Input: dimensioned drawing with shaded views. Units: mm. Origin: part minimum x, y, z. Give positions to 0.01 mm unless a question says otherwise; leave off trailing zeros. Order: outer loops, then holes, each group sorted by start corner. A loop starts at its lowest first (then second) coordinate and runs counter-clockwise, first axis right, second up. Notation, with made-up numbers: (27, 30) - (53, 30) arc R35 cw to (53, 69) - close; hole circle Ø4 at (-18.5, -22). An arc over 180 degrees is marked (long way). Answer as CSV lines item,"result".
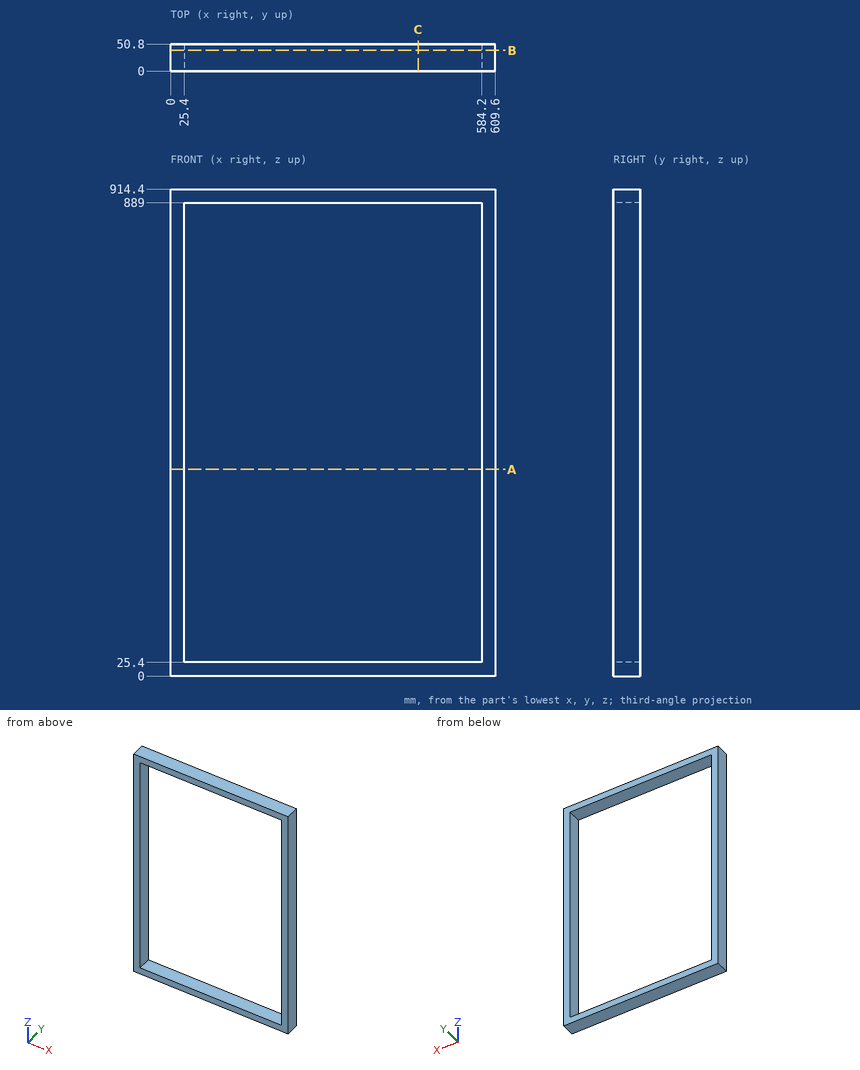
(1) Contact query for a flat-ended pin moving along its axis: pin 1 (1 mm diameter, centred on x = 237, y = 42.5, fed in from -Z). Output: stop coordinate, or through.
Completed:
pin 1,"z = 0"
(2) Cut plane C-C (x = 464.5). Return loops of the section in (y, z).
Completed:
outline,"(0, 0) - (50.8, 0) - (50.8, 25.4) - (0, 25.4) - close; (0, 889) - (50.8, 889) - (50.8, 914.4) - (0, 914.4) - close"
(3) Cut plane B-B (y = 39). Return loops of the section in (x, z).
Completed:
outline,"(0, 0) - (609.6, 0) - (609.6, 914.4) - (0, 914.4) - close; hole (25.4, 25.4) - (584.2, 25.4) - (584.2, 889) - (25.4, 889) - close"
(4) Ray query, line 1 (Z direction, x = 361.5, y = 45.5); line 2 (X direction, y = 3.5, z = 733.5). Return the intervals inside material, ascending. Write a range as from..to.
Completed:
line 1,"0..25.4, 889..914.4"
line 2,"0..25.4, 584.2..609.6"
(5) Cut plane A-A (z = 388). Return loops of the section in (x, y).
Completed:
outline,"(0, 0) - (25.4, 0) - (25.4, 50.8) - (0, 50.8) - close; (584.2, 0) - (609.6, 0) - (609.6, 50.8) - (584.2, 50.8) - close"
